Read the model definition and answer for the solid it produces. Units are mm, in the model's axes. A direction names the side the tool comes from. Coordinates: 2 decimals unless noted, no trailing zeros. Order: outer loops, then holes, each group sorted by start corner. A loop starts at its lowest first (then second) coordinate and runs counter-clockwise, first axis right, second up. Notation, with made-up numbers: M 57,50.5 L 104,50.5 A7 ccw 104,61.5 Z; hole C 6,71.5 d1. An arc over 180 degrees is marked long. Use a Markdown table: item, result. Add a question column.
1) Each of these flat-tipped pins is pushed along its axis until it touches: pin 1 Ø22.5 at (x, z) = (81.32, 81.32) entering from -Y; pin 2 Ø3 at (x, y) = (-94.5, 20.5) entering from -Z; pin 3 Ø19.5 at (x, z) = (-50, 0) entering from +Y; pin 4 Ø6 at (x, y) = (64, 34.5) entering from +Z. Where does it stop, or does it pass through?
2) Find section B-B on x = -118.5. Write down the section's boundary in (y, z).
3) Find section A-A on x = 0. Write down the section's boundary in (y, z).
4) For faces 4 (the face through (3.755, 19.72, 103.077)), 5 (the face through (42.846, 17.395, -2.253)), determine the directions among +Z, -Z, +X, -X, +Y, -Y from which every point of the face is accessible in a straight line to the end or side of a thin tool.
5) The mould has two halves that part along X. Classify faces 1 (the face through (106.69, 19.72, -105.44)), 2 (the face through (33, 40, -95)), 3 (the face through (103.077, 19.72, -3.755)): released by +X, released by -X, zero draft, split by the parting line, or undercut.
6) Find the intervals of material crossed by probe 1 along X at (y, z) = (28, 4.5); probe 2 along Z at (x, y) = (74.5, 10.5); probe 3 along Z at (x, y) = (-50, 16), in increasing order. Write a range as [from, to].
7) Find section C-C on y = 20. Count the separate pieces of the cut face and the enclosed holes in it, plus the area to 3 significant figures.
from build123d import *

# Parameters (mm, degrees)
SKETCH1_R                                = 150
BOSS_EXTRUDE1_DEPTH                      = 40
CBORE_FOR_M64_HEX_HEAD_BOLT1_D           = 75
CBORE_FOR_M64_HEX_HEAD_BOLT1_CBORE_D     = 175
CBORE_FOR_M64_HEX_HEAD_BOLT1_CBORE_DEPTH = 15
F_25_0_25_DIAMETER_HOLE1_D               = 25
CIRPATTERN2_COUNT                        = 8
CHAMFER1_SIZE                            = 12
CHAMFER1_SIZE2                           = 14.818765878
F_15_0_15_DIAMETER_HOLE1_D               = 15
F_15_0_15_DIAMETER_HOLE1_DEPTH           = 15
F_15_0_15_DIAMETER_HOLE1_TIP             = 4.506454643


with BuildPart() as part:
    # Sketch1 → Boss-Extrude1 (new body)
    with BuildSketch(Plane(origin=(0, 0, 0), x_dir=(1, 0, 0), z_dir=(0, 1, 0))):
        with Locations(Location((0, 0, 0), (0, 0, 270))):
            Circle(SKETCH1_R)
    extrude(amount=BOSS_EXTRUDE1_DEPTH)

    # CBORE for M64 Hex Head Bolt1 (through all)
    with Locations(Plane(origin=(0, 40, 0), x_dir=(1, 0, 0), z_dir=(0, 1, 0))):
        with Locations((0, 0)):
            CounterBoreHole(CBORE_FOR_M64_HEX_HEAD_BOLT1_D / 2, CBORE_FOR_M64_HEX_HEAD_BOLT1_CBORE_D / 2, CBORE_FOR_M64_HEX_HEAD_BOLT1_CBORE_DEPTH)

    # Ø25.0 (25) Diameter Hole1 (through all)
    with Locations(Plane(origin=(0, 40, 0), x_dir=(1, 0, 0), z_dir=(0, 1, 0))):
        with Locations((115, 0)):
            f_25_0_25_diameter_hole1 = Hole(F_25_0_25_DIAMETER_HOLE1_D / 2)

    # CirPattern2: Ø25.0 (25) Diameter Hole1 ×8 about axis
    cirpattern2_axis = Axis((0, 0, 0), (0, 1, 0))
    for i in range(1, CIRPATTERN2_COUNT):
        add(f_25_0_25_diameter_hole1.rotate(cirpattern2_axis, i * 360 / CIRPATTERN2_COUNT), mode=Mode.SUBTRACT)

    # Chamfer1
    chamfer1_edges = [part.edges().sort_by_distance(p)[0] for p in [
        (-87.5, 40, 0),
    ]]
    chamfer1_side = [part.faces().sort_by_distance(p)[0] for p in [
        (0, 40, -145.757359313),
    ]]
    chamfer(chamfer1_edges, length=CHAMFER1_SIZE, length2=CHAMFER1_SIZE2, reference=chamfer1_side[0])

    # SurfaceCut1
    split(bisect_by=Plane(origin=(-140, 0, 0), x_dir=(0, 0, -1), z_dir=(1, 0, 0)), keep=Keep.TOP)

    # SurfaceCut2
    split(bisect_by=Plane.XY.offset(140), keep=Keep.BOTTOM)

    # SurfaceCut3
    split(bisect_by=Plane(origin=(140, 0, 0), x_dir=(0, 0, -1), z_dir=(1, 0, 0)), keep=Keep.BOTTOM)

    # SurfaceCut4
    split(bisect_by=Plane.XY.offset(-140), keep=Keep.TOP)

    # Ø15.0 (15) Diameter Hole1
    with Locations(Plane(origin=(0, 25, 0), x_dir=(1, 0, 0), z_dir=(0, 1, 0))):
        with Locations((-50, 0), (50, 0)):
            Hole(F_15_0_15_DIAMETER_HOLE1_D / 2, depth=F_15_0_15_DIAMETER_HOLE1_DEPTH)
            with Locations((0, 0, -(F_15_0_15_DIAMETER_HOLE1_DEPTH + F_15_0_15_DIAMETER_HOLE1_TIP / 2))):  # 118° drill point
                Cone(0, F_15_0_15_DIAMETER_HOLE1_D / 2, F_15_0_15_DIAMETER_HOLE1_TIP, mode=Mode.SUBTRACT)


solid = part.part
Check result:
| question | item | result |
|---|---|---|
| 1 | pin 1 | passes through |
| 1 | pin 2 | stops at z = -117.69 |
| 1 | pin 3 | stops at y = 25 |
| 1 | pin 4 | stops at z = 137.04 |
| 2 | outline | M 0,-91.97 L 40,-91.97 L 40,-12 L 0,-12 Z; M 0,12 L 40,12 L 40,91.97 L 0,91.97 Z |
| 3 | outline | M 0,-140 L 40,-140 L 40,-127.5 L 0,-127.5 Z; M 0,-102.5 L 40,-102.5 L 40,-99.5 L 25.18,-87.5 L 25,-87.5 L 25,-37.5 L 0,-37.5 Z; M 0,37.5 L 25,37.5 L 25,87.5 L 25.18,87.5 L 40,99.5 L 40,102.5 L 0,102.5 Z; M 0,127.5 L 40,127.5 L 40,140 L 0,140 Z |
| 4 | face 4 | +Y, -Y |
| 4 | face 5 | +Y |
| 5 | face 1 | released by +X |
| 5 | face 2 | zero draft |
| 5 | face 3 | undercut |
| 6 | probe 1 | x = [-140, -126.66], [-103.34, -89.67], [89.67, 103.34], [126.66, 140] |
| 6 | probe 2 | z = [-130.19, -91.79], [-70.84, 70.84], [91.79, 130.19] |
| 6 | probe 3 | z = [-140, -7.5], [7.5, 140] |
| 7 | separate pieces | 1 |
| 7 | enclosed holes | 11 |
| 7 | area | 59,100 mm2 |
